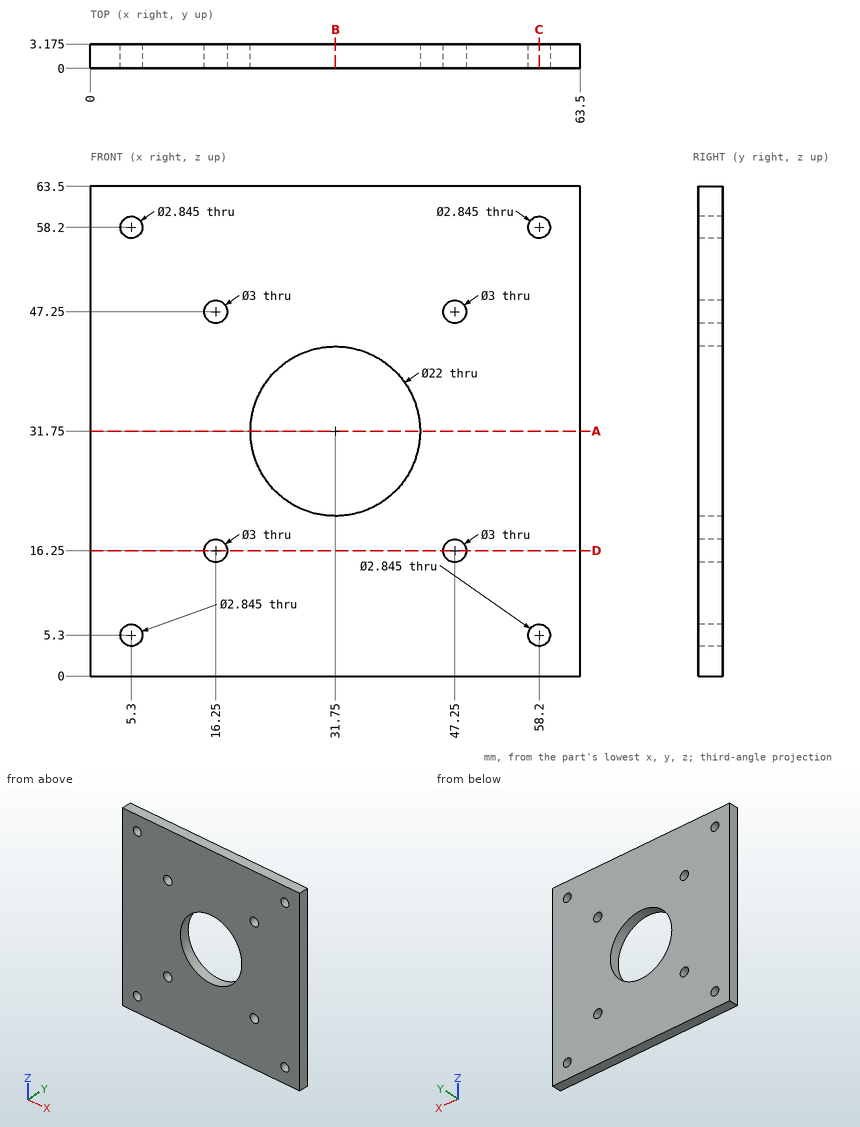
Could you check a few things on this drawing? It's one solid part, dimensions in mm from its lowest x, y, z. Round coordinates to 2 decimals unless told otherwise and drop trailing zeros. Write each loop counter-clockwise with the first axis right and the second up, starting at its lowest first coordinate (ties: lowest second). Pieces come first, ordered by that corner, then holes. Notation, with made-up numbers: M 48.5,56.25 L 98.5,56.25 A17 ccw 98.5,76.25 Z; hole C 1,62.5 d5. An arc over 180 degrees is marked long. Answer as CSV lines item,"result". Start each with the question number.
1. I'm going to push flat-ended pins straight in: pin 1 Ø2.5 at (x, z) = (5.3, 58.2) entering from -Y; pin 2 Ø3.5 at (x, z) = (58.2, 58.2) entering from +Y (3 decimals). Where does each tip first touch, or does it pass through?
2. Suppose I cut it at D-D on z = 16.25. Write out the boundary of the cut face in (x, y) (3 decimals).
3. I need wall thicknesses on probe 1 along Z at (x, y) = (5.3, 1.15); probe 2 along Z at (x, y) = (47.25, 2.5). Which ranges of each line are inside material? Lowest first, please.
4. Suppose I cut it at C-C on x = 58.2. Write out the boundary of the cut face in (y, z) (1 decimal).
5. Suppose I cut it at B-B on x = 31.75. Write out the boundary of the cut face in (y, z) (3 decimals).
6. Suppose I cut it at A-A on z = 31.75. Write out the boundary of the cut face in (x, y) (3 decimals), then the cut area to 3 significant figures.
Check result:
1,pin 1,"passes through"
1,pin 2,"stops at y = 3.175"
2,outline,"M 0,0 L 14.75,0 L 14.75,3.175 L 0,3.175 Z; M 17.75,0 L 45.75,0 L 45.75,3.175 L 17.75,3.175 Z; M 48.75,0 L 63.5,0 L 63.5,3.175 L 48.75,3.175 Z"
3,probe 1,"z = 0 to 3.88, 6.72 to 56.78, 59.62 to 63.5"
3,probe 2,"z = 0 to 14.75, 17.75 to 45.75, 48.75 to 63.5"
4,outline,"M 0,0 L 3.2,0 L 3.2,3.9 L 0,3.9 Z; M 0,6.7 L 3.2,6.7 L 3.2,56.8 L 0,56.8 Z; M 0,59.6 L 3.2,59.6 L 3.2,63.5 L 0,63.5 Z"
5,outline,"M 0,0 L 3.175,0 L 3.175,20.75 L 0,20.75 Z; M 0,42.75 L 3.175,42.75 L 3.175,63.5 L 0,63.5 Z"
6,outline,"M 0,0 L 20.75,0 L 20.75,3.175 L 0,3.175 Z; M 42.75,0 L 63.5,0 L 63.5,3.175 L 42.75,3.175 Z"
6,area,"132 mm2"
